Design review of the part built by this model. Coordinates are the model's own, in mm. A direction names the side the tool comes from. Coordinates: 2 decimals unless noted, no trailing zeros. Write each loop counter-clockwise with the first axis right and the second up, starting at its lowest first coordinate (ties: lowest second). Pieces come first, ordered by that corner, then holes.
Q1. Take a section at A-A, the plane z = 25.5. Write out the cut boundary in (x, y).
Q2. For pin 1 Ø1.5 at (x, z) = (168.5, 14.5) entering from -Y; pin 2 Ø4 at (x, y) = (143, 15.5) entering from -Z; pin 3 Ø4 at (x, y) = (359.5, 16.5) entering from +Z, all flat-tipped, find the tip position at first contact; note any pin that passes through.
Q3. For L1, parallel to Y at x = 78.5, z = -21; L2, parallel to Y at x = 442.5, z = 17, list the stretches that pass through material, from the lowest coordinate up.
Q4. The part is to be moulded in two halves that separate along Z. For faces 6 (the flat face through (500, 0, 0)), 7 (the flat face through (246, 15, 20.8)), 8 (the flat face through (246, 20.8, 15)), say which applies: released by +Z, released by -Z, zero draft, split by the parting line, or undercut.
Q5. For faces 1 (the flat face through (246, -10.9, -25)), 2 (the flat face through (246, 19.1, 25)), 3 (the flat face through (246, -20.8, 15)), 4 (the flat face through (246, 0, 30)), 5 (the flat face through (246, 25, 19.1)), list the 3-axis set-ups (+Z, -Z, +X, -X, +Y, -Y) from which the entire face can be reached by the end or side of a thin tool; tool diameter is ignored.
Q6. Take a section at C-C, the plane z = -15. Write out the cut boundary in (x, y).
from build123d import *

# Parameters (mm, degrees)
SKETCH_1_W          = 60
SKETCH_1_H          = 60
EXTRUDE_1_DEPTH     = 500
SKETCH_2_W          = 8.2
SKETCH_2_H          = 9.2
SKETCH_2_W_2        = 9.2
SKETCH_2_H_2        = 8.2
CUT_EXTRUDE_1_DEPTH = 501


with BuildPart() as part:
    # 草图1 → 凸台-拉伸1 (new body)
    with BuildSketch(Plane(origin=(0, 0, 0), x_dir=(0, 0, -1), z_dir=(1, 0, 0))):
        Rectangle(SKETCH_1_W, SKETCH_1_H)
    extrude(amount=EXTRUDE_1_DEPTH)

    # 草图2 → 切除-拉伸1 (cut, through all)
    with BuildSketch(Plane.ZY):
        with Locations((-15, 25.4)):
            Rectangle(SKETCH_2_W, SKETCH_2_H)
        with Locations((-15, -25.4)):
            Rectangle(SKETCH_2_W, SKETCH_2_H)
        with Locations((15, -25.4)):
            Rectangle(SKETCH_2_W, SKETCH_2_H)
        with Locations((15, 25.4)):
            Rectangle(SKETCH_2_W, SKETCH_2_H)
        with Locations((-25.4, 15)):
            Rectangle(SKETCH_2_W_2, SKETCH_2_H_2)
        with Locations((-25.4, -15)):
            Rectangle(SKETCH_2_W_2, SKETCH_2_H_2)
        with Locations((25.4, -15)):
            Rectangle(SKETCH_2_W_2, SKETCH_2_H_2)
        with Locations((25.4, 15)):
            Rectangle(SKETCH_2_W_2, SKETCH_2_H_2)
    extrude(amount=-CUT_EXTRUDE_1_DEPTH, mode=Mode.SUBTRACT)


solid = part.part
Responses:
1. outline: (0, -30) - (500, -30) - (500, -19.1) - (0, -19.1) - close; (0, -10.9) - (500, -10.9) - (500, 10.9) - (0, 10.9) - close; (0, 19.1) - (500, 19.1) - (500, 30) - (0, 30) - close
2. pin 1: stops at y = -20.8
2. pin 2: stops at z = -20.8
2. pin 3: stops at z = 20.8
3. L1: y = -30 to -19.1, -10.9 to 10.9, 19.1 to 30
3. L2: y = -20.8 to 20.8
4. face 6: zero draft
4. face 7: released by +Z
4. face 8: undercut
5. face 1: -Z, +X, -X
5. face 2: +Z, +X, -X
5. face 3: +X, -X, -Y
5. face 4: +Z, +X, -X, +Y, -Y
5. face 5: +X, -X, +Y
6. outline: (0, -20.8) - (500, -20.8) - (500, 20.8) - (0, 20.8) - close
